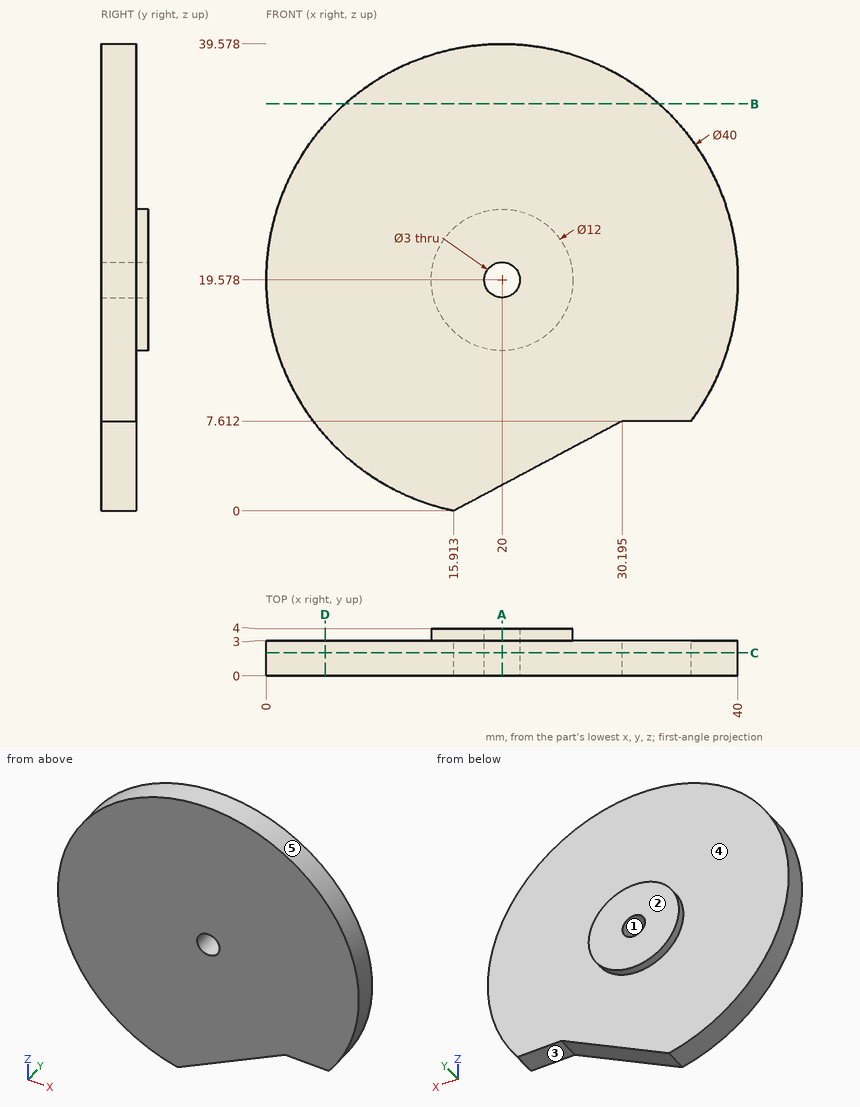
Drawing for the job (mm, zero at the part's lowest x, y, z). A direction names the side the tool comes from. Give positions to 0.01 mm unless a question says otherwise; leave off trailing zeros. Order: outer loops, then holes, each group sorted by start corner. A loop starts at its lowest first (then second) coordinate and runs counter-clockwise, first axis right, second up. Notation, with made-up numbers: M 76,38 L 112,38 A19 ccw 112,51 Z; hole C 89,40 d7. An arc over 180 degrees is marked long. Use a Markdown table: item, result. Add a question column.
(1) Saw through at A-A, the plane x = 20. Give the cut face in (y, z), and give its area (3 significant figures).
(2) Saw through at C-C, the plane y = 1.95. Give the cut face in (x, z) (1 decimal), and give its area (3 significant figures).
(3) Saw through at B-B, the plane z = 34.5. Give the cut face in (x, y).
(4) 3-axis set-ups, long thin cutter, end or side, ignore diameter. For the marked faces 4 and 5: which of +Z, -Z, +X, -X, +Y, -Y reach the whole face in a straight line?
(5) Drop flat-ended pins along their axis: P1, Ø1.5, axis at x = 4, y = 2, coming from the +Z side; P2, Ø2, axis at y = 1.5, z = 13.5, coming from the -X side (1 decimal); P3, Ø1, axis at x = 7.5, y = 2.5, coming from the +Z side. Give the stop position or say it passes through.
(6) Mould opens along Z. For the marked faces 1, 2 and 3 say: +Z half, -Z half, draft (parallel to the pull), parting line (faces both ways), or undercut.
(7) Probe line 1 along Y through (x, z) = (31.5, 9); line 2 along Z through (x, y) = (19, 2.25) (1 decimal); line 3 along Z through (x, y) = (20, 2.95). List the from-to ranges inside material, lowest first. Write a range as [from, to].
(8) Saw through at D-D, the plane x = 5. Give the cut face in (y, z).
Answer key:
| question | item | result |
|---|---|---|
| 1 | outline | M 0,2.18 L 3,2.18 L 3,13.58 L 4,13.58 L 4,18.08 L 0,18.08 Z; M 0,21.08 L 4,21.08 L 4,25.58 L 3,25.58 L 3,39.58 L 0,39.58 Z |
| 1 | area | 112 mm^2 |
| 2 | outline | M 15.9,0 L 30.2,7.6 L 36,7.6 A20 ccw long Z; hole C 20,19.6 d3 |
| 2 | area | 1,180 mm^2 |
| 3 | outline | M 6.68,0 L 33.32,0 L 33.32,3 L 6.68,3 Z |
| 4 | face 4 | +Y |
| 4 | face 5 | +Y, -Y |
| 5 | P1 | z = 32.52 |
| 5 | P2 | x = 0.7 |
| 5 | P3 | z = 35.58 |
| 6 | face 1 | undercut |
| 6 | face 2 | draft |
| 6 | face 3 | -Z half |
| 7 | line 1 | [0, 3] |
| 7 | line 2 | [1.6, 18.5], [20.7, 39.6] |
| 7 | line 3 | [2.18, 18.08], [21.08, 39.58] |
| 8 | outline | M 0,6.35 L 3,6.35 L 3,32.81 L 0,32.81 Z |
